Autodesk Inventor part; units mm, degrees
ref_plane "YZ Plane" through (0, 0, 0) normal (1, 0, 0) x (0, 1, 0)
ref_plane "XZ Plane" through (0, 0, 0) normal (0, 1, 0) x (-1, 0, 0)
ref_plane "XY Plane" through (0, 0, 0) normal (0, 0, 1) x (1, 0, 0)
sketch "Эскиз1" plane through (0, 0, 0) normal (0, 0, 1) x (1, 0, 0)
  circle A0 centre (0, 0) radius 1.5
  circle A1 centre (0, 0) radius 2.75
  dimension "d0" = 5.5
  dimension "d1" = 3
extrude "Выдавливание1" add sketch "Эскиз1" along normal blind 12 contours A0
extrude "Выдавливание2" add sketch "Эскиз1" against normal blind 1.5 contours A0 | A1
thread "Резьба1"
sketch "Эскиз2" plane through (0, 0, -1.5) normal (0, 0, -1) x (-1, 0, 0)
  line L0 (0, 1.1547) -> (1, 0.5774)
  line L1 (1, 0.5774) -> (1, -0.5774)
  line L2 (1, -0.5774) -> (0, -1.1547)
  line L3 (0, -1.1547) -> (-1, -0.5774)
  line L4 (-1, -0.5774) -> (-1, 0.5774)
  line L5 (-1, 0.5774) -> (0, 1.1547)
  point P0 (0, 0)
  point P1 (0, 0)
  dimension "d8" = 2
extrude "Выдавливание3" cut sketch "Эскиз2" against normal blind 1
fillet "Сопряжение1" radius 1 1 edges at (-2.75, 0, -1.5)
properties part number "Болт М3"
Could you check a few things on this model? Use its own coordinates, in mm. A direction names the side the tool comes from. Give positions to 0.01 mm unless a question says otherwise; leave off trailing zeros. Order: outer loops, then holes, each group sorted by start corner. A loop starts at its lowest first (then second) coordinate and runs counter-clockwise, first axis right, second up. Notation, with made-up numbers: (-40, -30) - (-1, -30) arc R32 cw to (-1, 6) - close; hole circle Ø6 at (59.25, 88.5). An arc over 180 degrees is marked (long way). One line per item, written item: value. Start each with the question number.
1. If I drill on probe 1 along Y at (x, z) = (0, 11); probe 2 along Y at (x, z) = (0.8, -0.75); probe 3 along Z at (x, y) = (-1.1, -1.25), over which ranges is the centre line in solid material (lowest first)?
2. Imagine slicing it at A-A on y = 0. List the corners of the cut face in (x, z) for me.
3. Thinking about a two-plate mould opening in Y: for faces 3 (the face through (-0.49, 0.87, -1.01)), 4 (the face through (1.2, -1.2, 0)), 5 (the face through (-1.5, -0.07, 5.92)), which applies, +Y half, -Y half, draft (parallel to the pull), parting line (faces both ways), or undercut?
4. For faces 1 (the face through (0, 0, -0.5)), 2 (the face through (0, 0, 12)), which set-ups out of +Z, -Z, +X, -X, +Y, -Y let a thin tool reach every point of the face, with its end or its side?
5. Imagine slicing it at B-B on z = 4.25. List the corners of the cut face in (x, y) for me.
6. For P1, Ø0.5, axis at y = 0, z = -1, coming from the -X side; P2, Ø3, axis at x = 1, z = 4.5, coming from the -Y side; P3, Ø1.5, axis at y = -1.5, z = 3.5, coming from the -X side; P4, Ø1.6, axis at x = 0.5, y = -0.5, coming from the -Z side, each with a flat end and sliding along its axis, tell me the tip position at first contact or that it passes through.
Values:
1. probe 1: -1.5 to 1.5
1. probe 2: -2.6 to -0.69, 0.69 to 2.6
1. probe 3: -1.5 to 0
2. outline: (-2.75, -0.5) arc R1 ccw to (-1.75, -1.5) - (-1, -1.5) - (-1, -0.5) - (1, -0.5) - (1, -1.5) - (1.75, -1.5) arc R1 ccw to (2.75, -0.5) - (2.75, 0) - (1.5, 0) - (1.5, 12) - (-1.5, 12) - (-1.5, 0) - (-2.75, 0) - close
3. face 3: undercut
3. face 4: draft
3. face 5: parting line
4. face 1: -Z
4. face 2: +Z, +X, -X, +Y, -Y
5. outline: circle Ø3 at (0, 0)
6. P1: x = -2.72
6. P2: y = -1.5
6. P3: x = -1.3
6. P4: z = -1.5
